Autodesk Inventor part; units mm, degrees
ref_plane "YZ Plane" through (0, 0, 0) normal (1, 0, 0) x (0, 1, 0)
ref_plane "XZ Plane" through (0, 0, 0) normal (0, 1, 0) x (-1, 0, 0)
ref_plane "XY Plane" through (0, 0, 0) normal (0, 0, 1) x (1, 0, 0)
sketch "Sketch1" plane through (0, 0, 0) normal (0, 1, 0) x (-1, 0, 0)
  line L0 (0, 0) -> (76.2, 0)
  line L1 (76.2, 0) -> (76.2, -25.4)
  line L2 (76.2, -25.4) -> (0, -25.4)
  line L3 (0, -25.4) -> (0, 0)
  dimension "d0" = 25.4
  dimension "d1" = 76.2
extrude "Extrusion1" add sketch "Sketch1" along normal blind 5
sketch "Sketch2" plane through (0, 0, 0) normal (1, 0, 0) x (0, 0, -1)
  line L0 (25.4, 0) -> (0, 0)
  line L1 (25.4, 0) -> (25.4, 5)
  line L2 (0, 5) -> (25.4, 5)
  line L3 (0, 0) -> (0, 5)
  line L4 (5.2, 0) -> (20.2, 0)
  line L5 (20.2, 0) -> (20.2, 5)
  line L6 (20.2, 5) -> (5.2, 5)
  line L7 (5.2, 5) -> (5.2, 0)
  dimension "d4" = 15
  dimension "d5" = 25.4
  dimension "d6" = 5.2
extrude "Extrusion2" add sketch "Sketch2" along normal blind 50.8 contours L0 L7 L2 L5
sketch "Sketch4" plane through (0, 5, 0) normal (0, 1, 0) x (1, 0, 0)
  circle A0 centre (-38.1, 12.7) radius 6.35
  line L0 (0, 20.2) -> (0, 25.4)
  line L1 (-76.2, 0) -> (0, 0)
  dimension "d12" = 12.7
  dimension "d13" = 38.1
  dimension "d14" = 12.7
extrude "Extrusion4" cut sketch "Sketch4" against normal blind 50.8
equation "\"d6\" = -0.5 * d4 + 0.5 * d5"
properties part number "TSV+In" material "Steel"
The listing builds one solid part. Answer for the finished solid, in the listing's coordinates (mm). A direction names the side the tool comes from. Round coordinates to 2 decimals unless told otherwise and drop trailing zeros. Order: outer loops, then holes, each group sorted by start corner. A loop starts at its lowest first (then second) coordinate and runs counter-clockwise, first axis right, second up. Notation, with made-up numbers: (-32.75, 36.5) - (4.25, 36.5) arc R24 ccw to (4.25, 66.5) - close; hole circle Ø8 at (18, 30.5). An arc over 180 degrees is marked (long way). Write item = value, one per line. Start each with the question number.
1) Section D-D, the plane z = -4 is taken. Write down the section's boundary in (x, y).
2) For a pull along Z with two mould halves and no side action, classify faces 4 (the flat face through (25, 3, -5.2)), 5 (the cylindrical face through (-34.686, 2.535, -18.054)), 6 (the flat face through (25, 2, -20.2)), 7 (the flat face through (-26, 5, -13)) as released by +Z, released by -Z, zero draft, split by the parting line, or undercut.
3) Section A-A, the plane z = -12.7 is taken. Write down the section's boundary in (x, y).
4) For faces 1 (the flat face through (50.8, 3, -13)), 2 (the flat face through (0, 2, -3)), 3 (the flat face through (0, 2, -23)), determine the directions among +Z, -Z, +X, -X, +Y, -Y from which every point of the face is accessible in a straight line to the end or side of a thin tool.
5) Section C-C, the plane x = -38.1 is taken. Write down the section's boundary in (y, z), plus the area to 3 significant figures.
6) Straight lines are drawn through the part: L1, parallel to X at y = 3.1, z = -12.7; L2, parallel to Z at x = -38.1, y = 1.9; L3, parallel to X at y = 4.5, z = -4.5. For each, find the intervals that lie inside material, in ascending order.
7) Given pin 1 (1.5 mm diameter, centred on y = 1.5, z = -2, fed in from +X); pin 2 (2.5 mm diameter, centred on x = 25, y = 1.5, fed in from +Z); pin 3 (1 mm diameter, centred on x = 28, y = 4, fed in from -Z), each flat-ended and moving along its own axis, determine where each tip first touches the part or whether it passes through.
8) Section B-B, the plane y = 4.2 is taken. Write down the section's boundary in (x, z), plus the area to 3 significant figures.
Results list:
q1.outline = (-76.2, 0) - (0, 0) - (0, 5) - (-76.2, 5) - close
q2.face_4 = released by +Z
q2.face_5 = undercut
q2.face_6 = released by -Z
q2.face_7 = zero draft
q3.outline = (-76.2, 0) - (-44.45, 0) - (-44.45, 5) - (-76.2, 5) - close; (-31.75, 0) - (50.8, 0) - (50.8, 5) - (-31.75, 5) - close
q4.face_1 = +Z, -Z, +X, +Y, -Y
q4.face_2 = +Z, +X, +Y, -Y
q4.face_3 = -Z, +X, +Y, -Y
q5.outline = (0, -25.4) - (5, -25.4) - (5, -19.05) - (0, -19.05) - close; (0, -6.35) - (5, -6.35) - (5, 0) - (0, 0) - close
q5.area = 63.5 mm^2
q6.L1 = -76.2 to -44.45, -31.75 to 50.8
q6.L2 = -25.4 to -19.05, -6.35 to 0
q6.L3 = -76.2 to 0
q7.pin_1 = 0
q7.pin_2 = -5.2
q7.pin_3 = -20.2
q8.outline = (-76.2, -25.4) - (0, -25.4) - (0, -20.2) - (50.8, -20.2) - (50.8, -5.2) - (0, -5.2) - (0, 0) - (-76.2, 0) - close; hole circle Ø12.7 at (-38.1, -12.7)
q8.area = 2,570 mm^2
